from build123d import *

# Parameters (mm, degrees)
CHANFREIN1_SIZE = 1


with BuildPart() as part:
    # Esquisse1 → Révolution1 (revolve)
    with BuildSketch(Plane.XY, mode=Mode.PRIVATE) as r_volution1_sk:
        Polygon((0, 1.5), (15, 1.5), (15, 0), (26, 0), (26, 2.5), (7.5, 2.5), (7.5, 7), (5, 7), (5, 5), (0, 5), align=None)
    revolve(r_volution1_sk.sketch.rotate(Axis((-19.163170338, 0, 0), (1, 0, 0)), 90), axis=Axis((-19.163170338, 0, 0), (1, 0, 0)))

    # Chanfrein1
    chanfrein1_edges = [part.edges().sort_by_distance(p)[0] for p in [
        (26, 0, -2.5),
    ]]
    chamfer(chanfrein1_edges, length=CHANFREIN1_SIZE)


solid = part.part
Build history of the part. All positions in model axes, mm. A direction names the side the tool comes from. Round coordinates to 2 decimals unless told otherwise and drop trailing zeros. Write each loop counter-clockwise with the first axis right and the second up, starting at its lowest first coordinate (ties: lowest second). Pieces come first, ordered by that corner, then holes. Notation, with made-up numbers: M 29.25,50.25 L 58.25,50.25 A28 ccw 58.25,80.25 Z; hole C 17.5,32.25 d7. An arc over 180 degrees is marked long. Use CSV: the item, a comma, the result in double quotes.
1. Saw through at A-A (z = 0). Give the cut face in (x, y), plus the area to 4 significant figures.
Reply:
outline,"M 0,-5 L 5,-5 L 5,-7 L 7.5,-7 L 7.5,-2.5 L 25,-2.5 L 26,-1.5 L 26,1.5 L 25,2.5 L 7.5,2.5 L 7.5,7 L 5,7 L 5,5 L 0,5 L 0,1.5 L 15,1.5 L 15,-1.5 L 0,-1.5 Z"
area,"131.5 mm²"
2. Saw through at C-C (x = 5.75). Give the cut face in (y, z), plus the area to 3 significant figures.
Reply:
outline,"C 0,0 d14; hole C 0,0 d3"
area,"147 mm²"
3. Tool access for faces 1 (the face through (5, -5, -2)), 2 (the face through (26, 0, 0)), 3 (the face through (7.5, 3, 0)): list every direction of +Z, -Z, +X, -X, +Y, -Y with a clear straight run to the whole face (end or side of a thin tool).
Reply:
face 1,"-X"
face 2,"+Z, -Z, +X, +Y, -Y"
face 3,"+X"
4. Saw through at D-D (z = 4.25). Give the cut face in (x, y), plus the area to 4 significant figures.
Reply:
outline,"M 0,-2.63 L 5,-2.63 L 5,-5.56 L 7.5,-5.56 L 7.5,5.56 L 5,5.56 L 5,2.63 L 0,2.63 Z"
area,"54.15 mm²"
5. Flat gauge pins, fed straight in: pin 1 (8 mm diameter, centred on x = 13.5, y = 0, fed in from +Z); pin 2 (1.5 mm diameter, centred on x = 9, y = 5.5, fed in from +Z) (3 decimals); pin 3 (3 mm diameter, centred on x = 2.5, y = -3.5, fed in from -Z); pin 4 (6 mm diameter, centred on x = 3.5, z = 3.5, fed in from -Y). Where does each tip first touch, or does it go through?
Reply:
pin 1,"stops at z = 2.5"
pin 2,"passes through"
pin 3,"stops at z = -4.58"
pin 4,"stops at y = -6.94"
6. Two-plate mould, pull along Y, no slides. Class faces 4 (the face through (7.6, -0.45, 1.43)), 5 (the face through (16.1, -0.1, -2.5)), 6 (the face through (0, -1.2, -1.2)), 7 (the face through (15, 0, 0)): +Y half, -Y half, draft (parallel to the pull), parting line (faces both ways), or undercut.
Reply:
face 4,"undercut"
face 5,"parting line"
face 6,"draft"
face 7,"undercut"
7. Wall check: probe 1 along Y at (x, z) = (4.25, 0); probe 2 along Y at (x, z) = (11.5, 0); probe 3 along X at (y, z) = (2.5, -3.5). Give the ranges that are in metal, low to high. Write a range as from..to.
Reply:
probe 1,"y = -5..-1.5, 1.5..5"
probe 2,"y = -2.5..-1.5, 1.5..2.5"
probe 3,"x = 0..7.5"
